Could you check a few things on this model? Use its own coordinates, in mm. A direction names the side the tool comes from. Give positions to 0.01 mm unless a question says otherwise; leave off trailing zeros. Order: outer loops, then holes, each group sorted by start corner. A loop starts at its lowest first (then second) coordinate and runs counter-clockwise, first axis right, second up. Notation, with made-up numbers: (55, 54) - (70, 54) arc R23 cw to (70, 70) - close; hole circle Ø5 at (25, 27.25). An arc over 180 degrees is marked (long way). Put each result on its own line as item: value.
Autodesk Inventor part; units mm, degrees
ref_plane "YZ Plane" through (0, 0, 0) normal (1, 0, 0) x (0, 1, 0)
ref_plane "XZ Plane" through (0, 0, 0) normal (0, 1, 0) x (-1, 0, 0)
ref_plane "XY Plane" through (0, 0, 0) normal (0, 0, 1) x (1, 0, 0)
sketch "Schizzo1" plane through (0, 0, 0) normal (0, 0, 1) x (1, 0, 0)
  line L0 (-8.5308, -2.9405) -> (22.4692, -2.9405)
  line L1 (22.4692, -2.9405) -> (22.4692, -1.7792)
  line L2 (22.4692, -1.7792) -> (16.2975, 7.0595)
  line L3 (-2.3591, 7.0595) -> (-8.5308, -1.7792)
  line L4 (-8.5308, -1.7792) -> (-8.5308, -2.9405)
  line L5 (6.9692, 7.0595) -> (6.9692, -2.9405)
  line L6 (6.9692, 7.0595) -> (27.9692, 7.0595) construction
  line L7 (27.9692, 7.0595) -> (23.9692, 7.0595) construction
  line L8 (23.9692, 7.0595) -> (23.9692, 3.0595) construction
  circle A0 centre (23.9692, 3.0595) radius 4 construction
  line L9 (6.9692, 7.0595) -> (-14.0308, 7.0595) construction
  line L10 (-14.0308, 7.0595) -> (-10.0308, 7.0595) construction
  line L11 (-10.0308, 7.0595) -> (-10.0308, 3.0595) construction
  circle A1 centre (-10.0308, 3.0595) radius 4 construction
  line L12 (-2.3591, 7.0595) -> (16.2975, 7.0595)
  dimension "d1" = 31
  dimension "d6" = 10
  dimension "d7" = 21
  dimension "d8" = 4
  dimension "d9" = 4
  dimension "d10" = 10
  dimension "d11" = 21
  dimension "d12" = 4
  dimension "d13" = 4
extrude "Estrusione1" add sketch "Schizzo1" along normal mid plane 105
sketch "Schizzo3" plane through (-2.3591, 7.0595, 52.5) normal (0, 1, 0) x (1, 0, 0)
  line L0 (18.6566, 0) -> (0, 0)
  line L1 (0, 52.5) -> (18.6566, 52.5) construction
  line L2 (18.6566, 0) -> (18.6566, 105)
  line L3 (0, 0) -> (9.3283, 0)
  line L4 (9.3283, 0) -> (9.3283, 105) construction
  line L5 (24.8283, 105) -> (-6.1717, 105)
  line L6 (9.3283, 92.5) -> (4.3283, 92.5)
  line L7 (4.3283, 92.5) -> (4.3283, 12.5)
  line L8 (4.3283, 12.5) -> (14.3283, 12.5)
  line L9 (14.3283, 12.5) -> (14.3283, 92.5)
  line L10 (14.3283, 92.5) -> (9.3283, 92.5)
  point P0 (2.3591, 52.5)
  dimension "d18" = 5
  dimension "d19" = 80
  dimension "d20" = 10
extrude "Estrusione2" cut sketch "Schizzo3" against normal blind 10
fillet "Raccordo1" radius 2 8 edges at (11.9692, 2.0595, 40) (1.9692, 2.0595, 40) (1.9692, 2.0595, -40) (11.9692, 2.0595, -40) (11.9692, 7.0595, 0) (1.9692, 7.0595, 0) (6.9692, 7.0595, -40) (6.9692, 7.0595, 40)
fillet "Raccordo2" radius 2 8 edges at (11.3834, -2.9405, -39.4142) (6.9692, -2.9405, -40) (2.555, -2.9405, -39.4142) (1.9692, -2.9405, 0) (2.555, -2.9405, 39.4142) (6.9692, -2.9405, 40) (11.3834, -2.9405, 39.4142) (11.9692, -2.9405, 0)
properties part number "esercizio3 02-27-2023"
1) If I drill on line 1 (Z direction, x = 8, y = 6); line 2 (X direction, y = -0.5, z = -18.5); line 3 (X direction, y = 3.25, z = -17.5), over which ranges is the centre line in solid material (lowest first)? Write a range as [from, to].
Filled in:
line 1: z = [-52.5, -40.23], [40.23, 52.5]
line 2: x = [-7.64, 1.97], [11.97, 21.58]
line 3: x = [-5.02, 1.97], [11.97, 18.96]
2) Suppose I cut it at B-B, the plane z = -34. List the corners of the cut face in (x, y) for me.
Filled in:
outline: (-8.53, -2.94) - (-0.03, -2.94) arc R2 ccw to (1.97, -0.94) - (1.97, 5.06) arc R2 ccw to (-0.03, 7.06) - (-2.36, 7.06) - (-8.53, -1.78) - close; (11.97, -0.94) arc R2 ccw to (13.97, -2.94) - (22.47, -2.94) - (22.47, -1.78) - (16.3, 7.06) - (13.97, 7.06) arc R2 ccw to (11.97, 5.06) - close
3) I'm going to push flat-ended pins straight in: pin 1 (3 mm diameter, centred on x = 11.5, z = -33, fed in from -Y); pin 2 (1.8 mm diameter, centred on y = 0.5, z = 12.5, fed in from -X); pin 3 (1.8 mm diameter, centred on y = 2.5, z = 15.5, fed in from +X). Where does each tip first touch, or does it pass through?
Filled in:
pin 1: stops at y = -2.69
pin 2: stops at x = -7.57
pin 3: stops at x = 20.11
4) Suppose I cut it at C-C, the plane y = 1. List the corners of the cut face in (x, z) for me, and give its area (3 significant figures).
Filled in:
outline: (-6.59, -52.5) - (20.53, -52.5) - (20.53, 52.5) - (-6.59, 52.5) - close; hole (1.97, -38) arc R2 ccw to (3.97, -40) - (9.97, -40) arc R2 ccw to (11.97, -38) - (11.97, 38) arc R2 ccw to (9.97, 40) - (3.97, 40) arc R2 ccw to (1.97, 38) - close
area: 2,050 mm^2
5) Which directions (+Z, -Z, +X, -X, +Y, -Y) give clear straight access to the entire face, cutting with the end or side of a thin tool? Please do faces 1 (the cylindrical face through (1.4, -2.34, -0.53)), 2 (the cylindrical face through (7.01, 6.49, -40.6)), 3 (the cylindrical face through (2.54, 2.02, -39.4)), 4 (the flat face through (7, 2, 52.5)), 5 (the flat face through (-4, -2.94, -1)).
Filled in:
face 1: -Y
face 2: +Y
face 3: +Y, -Y
face 4: +Z, +X, -X, +Y, -Y
face 5: +Z, -Z, +X, -X, -Y
6) Suppose I cut it at D-D, the plane z = -44.5. List the corners of the cut face in (x, y) for me, and give its area (3 significant figures).
Filled in:
outline: (-8.53, -2.94) - (22.47, -2.94) - (22.47, -1.78) - (16.3, 7.06) - (-2.36, 7.06) - (-8.53, -1.78) - close
area: 255 mm^2
7) Suppose I cut it at A-A, the plane x = 6. List the corners of the cut face in (y, z) for me.
Filled in:
outline: (-2.94, -52.5) - (7.06, -52.5) - (7.06, -42) arc R2 ccw to (5.06, -40) - (-0.94, -40) arc R2 ccw to (-2.94, -42) - close; (-2.94, 42) arc R2 ccw to (-0.94, 40) - (5.06, 40) arc R2 ccw to (7.06, 42) - (7.06, 52.5) - (-2.94, 52.5) - close
